```python
from build123d import *

# Parameters (mm, degrees)
CBORE_FOR_2_BINDING_HEAD_MACHINE_SCREW1_D           = 2.4384
CBORE_FOR_2_BINDING_HEAD_MACHINE_SCREW1_CBORE_D     = 5.55752
CBORE_FOR_2_BINDING_HEAD_MACHINE_SCREW1_CBORE_DEPTH = 5.269992


with BuildPart() as part:
    # Sketch13 → Revolve1 (revolve)
    with BuildSketch(Plane.XY, mode=Mode.PRIVATE) as revolve1_sk:
        with BuildLine():
            Line((0, -31.75), (-9.5, -31.75))
            ThreePointArc((-9.5, -31.75), (-5.964466094, -30.285533906), (-4.5, -26.75))
            Line((-4.5, -26.75), (-4.5, -17.526))
            Line((-4.5, -17.526), (0, -17.526))
            Line((0, -17.526), (0, -31.75))
        make_face()
    revolve(revolve1_sk.sketch.rotate(Axis((16.880780842, 0, 0), (-1, 0, 0)), 180), axis=Axis((16.880780842, 0, 0), (-1, 0, 0)))

    # CBORE for #2 Binding Head Machine Screw1 (through all)
    with Locations(Plane(origin=(-9.5, 0, 0), x_dir=(0, 0, -1), z_dir=(-1, 0, 0))):
        with Locations((-28.575, 0), (0, -28.575), (28.575, 0), (0, 28.575)):
            CounterBoreHole(CBORE_FOR_2_BINDING_HEAD_MACHINE_SCREW1_D / 2, CBORE_FOR_2_BINDING_HEAD_MACHINE_SCREW1_CBORE_D / 2, CBORE_FOR_2_BINDING_HEAD_MACHINE_SCREW1_CBORE_DEPTH)


solid = part.part
```
Model file for the job. Use its own axes, mm. A direction names the side the tool comes from. Round coordinates to 2 decimals unless told otherwise and drop trailing zeros. Loops run counter-clockwise (first coordinate to the right, second up) from the corner with the lowest first, then second, coordinate; pieces in that order, holes last. Notation, with made-up numbers: M -26,60.5 L 14,60.5 A25 cw 14,83.5 Z; hole C 41,43 d10. An arc over 180 degrees is marked long. Put each result on its own line as item: value. Start each with the question number.
Item 1: Mould opens along Z. For faces 1 (the face through (-4.23, 30, -1)), 2 (the face through (0, -14, 14)), 3 (the face through (-4.816, -6.883, 30.995)), 4 (the face through (-4.23, 1, 27)) say: released by +Z, released by -Z, zero draft, split by the parting line, or undercut.
Item 2: 3-axis set-ups, long thin cutter, end or side, ignore diameter. For faces 5 (the face through (-2.085, -0.366, 29.738)), 6 (the face through (-5.18, -0.12, 31.35)): which of +Z, -Z, +X, -X, +Y, -Y reach the whole face in a straight line?
Item 3: Drop flat-ended pins along their axis: P1, Ø2, axis at y = -1, z = 20, coming from the -X side; P2, Ø1, axis at x = -4, y = 0.5, coming from the +Z side; P3, Ø2, axis at x = -4.5, y = -18.5, coming from the +Z side. Give the stop position or say it passes through.
Item 4: Drill centre lines: line 1 along X through (y, z) = (13, -13); line 2 along Y through (x, z) = (-0.75, 1); line 3 along Z through (x, y) = (-7.25, 22). Where is each one in solid material? Low to high.
Item 5: Cut at A-A (y = 0). List the corners of the cut face in (x, z), then the cut area to 3 significant figures.
Answer block:
1. face 1: undercut
1. face 2: zero draft
1. face 3: split by the parting line
1. face 4: undercut
2. face 5: +X, -X
2. face 6: -X
3. P1: x = -4.5
3. P2: z = 31.75
3. P3: z = 26.49
4. line 1: -4.5 to 0
4. line 2: -31.73 to -29.27, -27.88 to -17.5, 17.5 to 27.88, 29.27 to 31.73
4. line 3: -22.89 to -22.14, 22.14 to 22.89
5. outline: M -9.5,-31.75 L 0,-31.75 L 0,-29.79 L -4.23,-29.79 L -4.23,-31.35 L -7.55,-31.35 A5 cw Z; M -9.5,31.75 A5 cw -7.55,31.35 L -4.23,31.35 L -4.23,29.79 L 0,29.79 L 0,31.75 Z; M -4.5,-25.8 L -4.23,-25.8 L -4.23,-27.36 L 0,-27.36 L 0,-17.53 L -4.5,-17.53 Z; M -4.5,17.53 L 0,17.53 L 0,27.36 L -4.23,27.36 L -4.23,25.8 L -4.5,25.8 Z
5. area: 107 mm2
